Could you check a few things on this model? Use its own coordinates, in mm. A direction names the side the tool comes from. Round coordinates to 2 decimals unless told otherwise and drop trailing zeros. Write each loop counter-clockwise with the first axis right and the second up, starting at its lowest first coordinate (ties: lowest second). Pieces come first, ordered by that corner, then holes. Notation, with made-up numbers: (46.25, 29) - (82.25, 29) arc R20 ccw to (82.25, 47) - close; hole circle Ø9 at (16, 31). An arc over 180 degrees is marked (long way). Put each result on its own line as item: value.
from build123d import *

# Parameters (mm, degrees)
BOSS_EXTRUDE1_DEPTH             = 15
M3X0_5_TAPPED_HOLE1_D           = 2.5
M3X0_5_TAPPED_HOLE1_CSINK_D     = 3.05
M3X0_5_TAPPED_HOLE1_CSINK_ANGLE = 90


with BuildPart() as part:
    # Sketch1 → Boss-Extrude1 (new body)
    with BuildSketch(Plane.XY):
        Polygon((-15, 0), (15, 0), (15, -10), (5, -10), (5, -5), (-5, -5), (-5, -10), (-15, -10), align=None)
    extrude(amount=BOSS_EXTRUDE1_DEPTH)

    # M3x0.5 Tapped Hole1 (through all)
    with Locations(Plane(origin=(0, 0, 0), x_dir=(1, 0, 0), z_dir=(0, 1, 0))):
        with Locations((0, -7.5)):
            CounterSinkHole(M3X0_5_TAPPED_HOLE1_D / 2, M3X0_5_TAPPED_HOLE1_CSINK_D / 2, counter_sink_angle=M3X0_5_TAPPED_HOLE1_CSINK_ANGLE)


solid = part.part
(1) Imagine slicing it at B-B, the plane z = 7.5. List the corners of the cut face in (x, y) for me (3 decimals), then the cut area to 3 significant figures.
Values found:
outline: (-15, -10) - (-5, -10) - (-5, -5) - (-1.25, -5) - (-1.25, -0.275) - (-1.525, 0) - (-15, 0) - close; (1.25, -5) - (5, -5) - (5, -10) - (15, -10) - (15, 0) - (1.525, 0) - (1.25, -0.275) - close
area: 237 mm^2
(2) Please list where these lines run through material, in increasing order: probe 1 along X at (y, z) = (-9, 4); probe 2 along Z at (x, y) = (0, -3.5); probe 3 along X at (y, z) = (-3.05, 7.5). Write a range as from..to.
Values found:
probe 1: x = -15..-5, 5..15
probe 2: z = 0..6.25, 8.75..15
probe 3: x = -15..-1.25, 1.25..15
(3) Imagine slicing it at D-D, the plane z = 3. List the corners of the cut face in (x, y) for me, then the cut area to 3 significant figures.
Values found:
outline: (-15, -10) - (-5, -10) - (-5, -5) - (5, -5) - (5, -10) - (15, -10) - (15, 0) - (-15, 0) - close
area: 250 mm^2
(4) Imagine slicing it at A-A, the plane x = 0. List the corners of the cut face in (y, z) for me (3 decimals).
Values found:
outline: (-5, 0) - (0, 0) - (0, 5.975) - (-0.275, 6.25) - (-5, 6.25) - close; (-5, 8.75) - (-0.275, 8.75) - (0, 9.025) - (0, 15) - (-5, 15) - close
(5) For faces 1 (the face through (-5, -7, 7)), 2 (the face through (0, -4, 0)), which set-ups out of +Z, -Z, +X, -X, +Y, -Y let a thin tool reach every point of the face, with its end or its side?
Values found:
face 1: +Z, -Z, -Y
face 2: -Z, +X, -X, +Y, -Y
(6) Imagine slicing it at C-C, the plane y = -9. List the corners of the cut face in (x, z) for me, then the cut area to 3 significant figures.
Values found:
outline: (-15, 0) - (-5, 0) - (-5, 15) - (-15, 15) - close; (5, 0) - (15, 0) - (15, 15) - (5, 15) - close
area: 300 mm^2
(7) If we mould it in two halves opening along X, with no side actions, what happens to faces 3 (the face through (15, -5, 7)), 4 (the face through (0, -5, 6)), 5 (the face through (-0.2, 0, 5.7))? For each: pulls with the +X half, pulls with the -X half, needs draft (parallel to the pull), parting line crosses it, or undercut.
Values found:
face 3: pulls with the +X half
face 4: undercut
face 5: needs draft
(8) I'm going to push flat-ended pins straight in: pin 1 (3 mm diameter, centred on x = 0, z = 7.5, fed in from +Y) (3 decimals); pin 2 (4 mm diameter, centred on x = -9.5, y = -3, fed in from -Z). Where does each tip first touch, or does it pass through?
Values found:
pin 1: stops at y = -0.025
pin 2: stops at z = 0
